from build123d import *

# Parameters (mm, degrees)
SKETCH253_W     = 12
SKETCH253_H     = 20
PAD126_DEPTH    = 1.3
SKETCH254_R     = 1.5
POCKET110_DEPTH = 3


with BuildPart() as part:
    # Sketch253 → Pad126 (new body)
    with BuildSketch(Plane(origin=(0, 0, -20), x_dir=(1, 0, 0), z_dir=(0, 0, -1))):
        with Locations((-11, 0)):
            Rectangle(SKETCH253_W, SKETCH253_H)
    extrude(amount=PAD126_DEPTH)

    # Sketch254 → Pocket110 (cut)
    with BuildSketch(Plane(origin=(0, 0, -20), x_dir=(1, 0, 0), z_dir=(0, 0, -1))):
        with Locations((-7, 8)):
            Circle(SKETCH254_R)
        with Locations((-7, -8)):
            Circle(SKETCH254_R)
    extrude(amount=POCKET110_DEPTH, mode=Mode.SUBTRACT)


with BuildPart() as part_1:
    # Body028 placement: moved
    add(part.part.moved(Location((-216, 0, -9))))


solid = part_1.part
Input: part model. Units: mm. Frame: model coordinates. Give positions to 0.01 mm unless a question says otherwise; leave off trailing zeros. Write each loop counter-clockwise with the first axis right and the second up, starting at its lowest first coordinate (ties: lowest second). Pieces come first, ordered by that corner, then holes. Notation, with made-up numbers: M -25.75,20.5 L 21.25,20.5 A24 ccw 21.25,30.5 Z; hole C -28.5,67 d3. An arc over 180 degrees is marked long. Use one line per item in the form item = value.
1. Cut plane D-D on y = 8.5. Return loops of the section in (x, z), and give its area (3 significant figures).
Outcome:
outline = M -233,-30.3 L -224.41,-30.3 L -224.41,-29 L -233,-29 Z; M -221.59,-30.3 L -221,-30.3 L -221,-29 L -221.59,-29 Z
area = 11.9 mm²
2. Cut plane A-A on x = -223. Return loops of the section in (y, z).
Outcome:
outline = M -10,-30.3 L -9.5,-30.3 L -9.5,-29 L -10,-29 Z; M -6.5,-30.3 L 6.5,-30.3 L 6.5,-29 L -6.5,-29 Z; M 9.5,-30.3 L 10,-30.3 L 10,-29 L 9.5,-29 Z
3. Cut plane C-C on z = -29.7. Return loops of the section in (x, y), and give its area (3 significant figures).
Outcome:
outline = M -233,-10 L -221,-10 L -221,10 L -233,10 Z; hole C -223,-8 d3; hole C -223,8 d3
area = 226 mm²
4. Ray query, L1, parallel to Y at x = -223, z = -29.5; L2, parallel to X at y = -8, z = -29.9; L3, parallel to Y at x = -224, z = -29.3. Return the intervals inside material, ascending.
Outcome:
L1 = -10 to -9.5, -6.5 to 6.5, 9.5 to 10
L2 = -233 to -224.5, -221.5 to -221
L3 = -10 to -9.12, -6.88 to 6.88, 9.12 to 10
5. Mould query, pull axis X, two halves, no side actions, for faces 1 (the face through (-221, 0, -30)), 2 (the face through (-221.614, -7.425, -29.641)), 3 (the face through (-227, 0, -29)). Classes: released by +X, released by -X, zero draft, split by the parting line, or undercut.
Outcome:
face_1 = released by +X
face_2 = undercut
face_3 = zero draft
6. Cut plane B-B on y = -8. Return loops of the section in (x, z).
Outcome:
outline = M -233,-30.3 L -224.5,-30.3 L -224.5,-29 L -233,-29 Z; M -221.5,-30.3 L -221,-30.3 L -221,-29 L -221.5,-29 Z
